from build123d import *

# Parameters (mm, degrees)
PAD_DEPTH   = 12
SKETCH001_R = 3
HOLE_DEPTH  = 25


with BuildPart() as part:
    # Sketch → Pad (new body)
    with BuildSketch(Plane.XY):
        Polygon((-20, -11.805553), (5, -11.805553), (5, -7.905553), (16, -7.905553), (16, -4.905553), (5, -5.355553), (5, -1.355553), (16, -1.805553), (16, 1.194447), (5, 1.194447), (0, 1.194447), (0, -8.805553), (-20, -8.805553), align=None)
    extrude(amount=PAD_DEPTH)

    # Sketch001 (on Face5 of Pad) → Hole (cut)
    with BuildSketch(Plane.XZ.offset(11.805553)):
        with Locations((-10, 6)):
            Circle(SKETCH001_R)
    extrude(amount=-HOLE_DEPTH, mode=Mode.SUBTRACT)


solid = part.part
Input: part model. Units: mm. Frame: model coordinates. A direction names the side the tool comes from. Round coordinates to 2 decimals unless told otherwise and drop trailing zeros. Loops run counter-clockwise (first coordinate to the right, second up) from the corner with the lowest first, then second, coordinate; pieces in that order, holes last. Notation, with made-up numbers: M 56.25,34 L 70.25,34 A28 ccw 70.25,61 Z; hole C -2.75,78.25 d8. An arc over 180 degrees is marked long. Answer as CSV lines item,"result". Start each with the question number.
(1) Section D-D, the plane y = -2.75. Output: boundary loops of the cut face in (x, z), plus the area to 3 significant figures.
(2) Section C-C, the plane z = 2. Output: boundary loops of the cut face in (x, y), plus the area to 3 significant figures.
(3) First-contact query: pin 1 (1.5 mm diameter, centred on y = -9, z = 9, fed in from +X); pin 2 (4 mm diameter, centred on y = 0, z = 10, fed in from -X). Flat tips, straight axial feed; report the tip coordinate or a pass-through.
(4) Line query: line 1 (Z direction, x = -10, y = -10.1); line 2 (X direction, y = -1, z = 1.25); line 3 (X direction, y = -4.75, z = 3). Output: solid intervals per line, ascending. Write a range as [from, to].
(5) Reachability of faces 4 (the flat face through (10, -7.906, 6)), 5 (the flat face through (16, 0, 6)), 6 (the flat face through (10.577, -5.127, 5.916)), 7 (the cylindrical face through (-12.4, -10.3, 4.2)), 8 (the flat face through (-12, -8.806, 3)) from +Z, -Z, +X, -X, +Y, -Y: full face, straight path, thin tool, end or side. Return the list, or none.
(6) Section B-B, the plane x = -10. Output: boundary loops of the cut face in (y, z), plus the area to 3 significant figures.
(7) Section A-A, the plane z = 6. Output: boundary loops of the cut face in (x, y).
(8) Draft query along Y for faces 1 (the flat face through (2, -7, 12)), 2 (the flat face through (10.423, -1.577, 5.916)), 3 (the flat face through (-5, -11.806, 6)). Return one class per face: released by +Y, released by -Y, zero draft, split by the parting line, or undercut.
Values found:
1,outline,"M 0,0 L 5,0 L 5,12 L 0,12 Z"
1,area,"60.0 mm²"
2,outline,"M -20,-11.81 L 5,-11.81 L 5,-7.91 L 16,-7.91 L 16,-4.91 L 5,-5.36 L 5,-1.36 L 16,-1.81 L 16,1.19 L 0,1.19 L 0,-8.81 L -20,-8.81 Z"
2,area,"186 mm²"
3,pin 1,"stops at x = 5"
3,pin 2,"stops at x = 0"
4,line 1,"z = [0, 3], [9, 12]"
4,line 2,"x = [0, 16]"
4,line 3,"x = [0, 5]"
5,face 4,"+Z, -Z, +X, -Y"
5,face 5,"+Z, -Z, +X, +Y, -Y"
5,face 6,"+Z, -Z"
5,face 7,"+Y, -Y"
5,face 8,"+Z, -Z, -X, +Y"
6,outline,"M -11.81,0 L -8.81,0 L -8.81,3 L -11.81,3 Z; M -11.81,9 L -8.81,9 L -8.81,12 L -11.81,12 Z"
6,area,"18.0 mm²"
7,outline,"M -20,-11.81 L -13,-11.81 L -13,-8.81 L -20,-8.81 Z; M -7,-11.81 L 5,-11.81 L 5,-7.91 L 16,-7.91 L 16,-4.91 L 5,-5.36 L 5,-1.36 L 16,-1.81 L 16,1.19 L 0,1.19 L 0,-8.81 L -7,-8.81 Z"
8,face 1,"zero draft"
8,face 2,"undercut"
8,face 3,"released by -Y"
